```python
from build123d import *

# Parameters (mm, degrees)
SKETCH001_W  = 317.5
SKETCH001_H  = 317.5
PAD001_DEPTH = 266.7
SKETCH_W     = 304.8
SKETCH_H     = 304.8
POCKET_DEPTH = 254.001
SKETCH002_W  = 304.8
SKETCH002_H  = 304.8
PAD_DEPTH    = 12.7


with BuildPart() as part:
    # Sketch001 → Pad001 (new body)
    with BuildSketch(Plane.XY):
        Rectangle(SKETCH001_W, SKETCH001_H)
    extrude(amount=PAD001_DEPTH)

    # Sketch → Pocket (cut, through all)
    with BuildSketch(Plane.XY.offset(12.7)):
        Rectangle(SKETCH_W, SKETCH_H)
    extrude(amount=POCKET_DEPTH, mode=Mode.SUBTRACT)

    # Sketch002 → Pad (join)
    with BuildSketch(Plane.XY):
        Rectangle(SKETCH002_W, SKETCH002_H)
    extrude(amount=-PAD_DEPTH)


solid = part.part
```
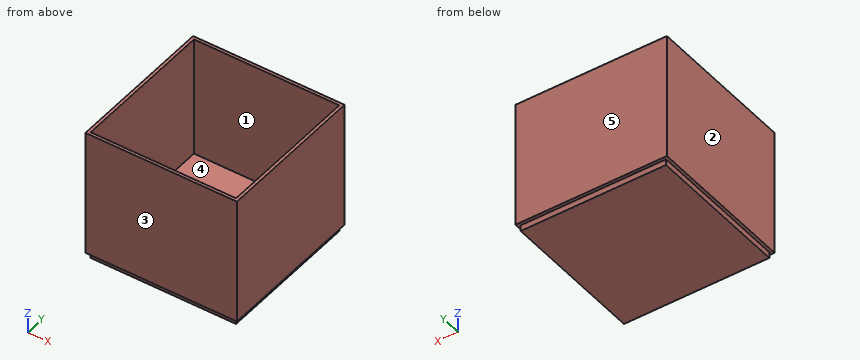
Input: part model. Units: mm. Frame: model coordinates. Face numbers are marked on the shaded views. A direction names the side the tool comes from. Give positions to 0.01 mm unless a question says otherwise; leave off trailing zeros. Loops run counter-clockwise (first coordinate to the right, second up) from the corner with the lowest first, then second, coordinate; pieces in that order, holes last. Notation, with made-up numbers: (51.25, -26) -> (82.25, -26) arc R8 ccw to (82.25, -21) -> close; hole circle Ø10 at (-16.75, -34.75). An arc over 180 degrees is marked (long way). Use a Markdown table: item, result.
Q1. Pull-direction query (Y, two-part tool) for the marked faces 1, 2 and 3; classes: pulls with the +Y half, pulls with the -Y half, needs draft (parallel to the pull), parting line crosses it, or undercut.
Entries:
| item | result |
|---|---|
| face 1 | undercut |
| face 2 | needs draft |
| face 3 | pulls with the -Y half |
Q2. Ray query, probe 1 along Y at (x, z) = (58, 188); probe 2 along Z at (x, y) = (128, 89). Return the intervals inside material, ascending. Write a range as from..to.
Entries:
| item | result |
|---|---|
| probe 1 | y = -158.75..-152.4, 152.4..158.75 |
| probe 2 | z = -12.7..12.7 |
Q3. Section query A-A, the plane z = 141. Return the cut outline in (x, y).
Entries:
| item | result |
|---|---|
| outline | (-158.75, -158.75) -> (158.75, -158.75) -> (158.75, 158.75) -> (-158.75, 158.75) -> close; hole (-152.4, -152.4) -> (152.4, -152.4) -> (152.4, 152.4) -> (-152.4, 152.4) -> close |
Q4. First-contact query: P1, Ø10, axis at x = -18.5, y = -115, coming from the +Z side; P2, Ø14, axis at x = -46.5, z = -7.5, coming from the +Y side. Flat tips, straight axial feed; report the tip coordinate or a pass-through.
Entries:
| item | result |
|---|---|
| P1 | stops at z = 12.7 |
| P2 | stops at y = 152.4 |
Q5. Section query B-B, the plane y = -65.5. Return the cut outline in (x, z).
Entries:
| item | result |
|---|---|
| outline | (-158.75, 0) -> (-152.4, 0) -> (-152.4, -12.7) -> (152.4, -12.7) -> (152.4, 0) -> (158.75, 0) -> (158.75, 266.7) -> (152.4, 266.7) -> (152.4, 12.7) -> (-152.4, 12.7) -> (-152.4, 266.7) -> (-158.75, 266.7) -> close |
Q6. Access query for the marked faces 4 and 5. Directions: +Z, -Z, +X, -X, +Y, -Y. A direction counts if a zero-diameter tool reaches every point of the face in a straight line with its end or side. Return the directions, or none.
Entries:
| item | result |
|---|---|
| face 4 | +Z |
| face 5 | +Z, -Z, +X, -X, +Y |
